Verification items for this drawing (mm, ordinates from the low corner). Coordinates: 2 decimals unless noted, no trailing zeros. Order: outer loops, then holes, each group sorted by start corner. A loop starts at its lowest first (then second) coordinate and runs counter-clockwise, first axis right, second up. Notation, with made-up numbers: M 35.25,30 L 91.25,30 A17 cw 91.25,62 Z; hole C -14,-40 d5. An arc over 180 degrees is marked long. Answer as a JSON object with one key per item and string values. Group by question number.
(1) Material ranges on line 1 (Z direction, x = 0.3, y = 78); line 2 (Z direction, x = 1.05, y = 45.5) (1 decimal); line 3 (Y direction, x = 1.3, z = 98), recorded low to high.
(2) Cross-section at D-D (y = 67.5). Enter the section's corners in (x, z).
(3) Cross-section at A-A (y = 122.5). Enter the section's corners in (x, z), plus the area to 3 significant figures.
(4) Cross-section at C-C (x = 0.6). Enter the section's corners in (y, z).
(5) Cross-section at B-B (z = 72.5). Enter the section's corners in (x, y).
(6) Gauge pin test, flat ends, axial feed: pin 1 Ø2 at (x, y) = (2.5, 65.5) entering from -Z; pin 2 Ø2 at (x, y) = (1, 64.5) entering from +Z; pin 3 Ø1 at (x, z) = (2, 47) entering from -Y. Record the tip position at first contact, or that the pin passes through.
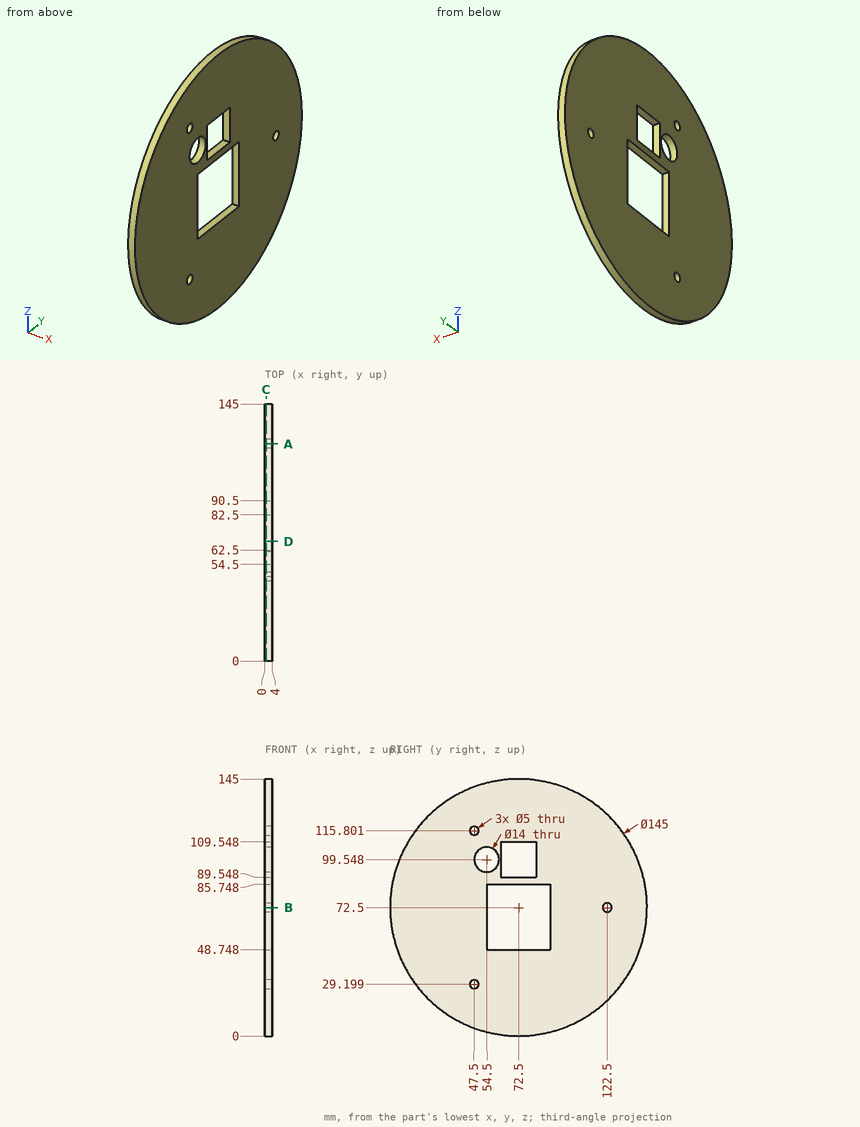
Taken from the geometry:
{
 "1": {"line 1": "z = 0.21 to 48.75, 85.75 to 89.55, 109.55 to 144.79", "line 2": "z = 5.2 to 27.7, 30.7 to 114.3, 117.3 to 139.8", "line 3": "y = 4.63 to 47.67, 61.33 to 62.5, 82.5 to 140.37"},
 "2": {"outline": "M 0,0.17 L 4,0.17 L 4,48.75 L 0,48.75 Z; M 0,85.75 L 4,85.75 L 4,89.55 L 0,89.55 Z; M 0,109.55 L 4,109.55 L 4,144.83 L 0,144.83 Z"},
 "3": {"outline": "M 0,20 L 4,20 L 4,70 L 0,70 Z; M 0,75 L 4,75 L 4,125 L 0,125 Z", "area": "400 mm²"},
 "4": {"outline": "C 72.5,72.5 d145; hole C 47.5,29.2 d5; hole C 47.5,115.8 d5; hole C 54.5,99.55 d14; hole M 54.5,48.75 L 90.5,48.75 L 90.5,85.75 L 54.5,85.75 Z; hole M 62.5,89.55 L 82.5,89.55 L 82.5,109.55 L 62.5,109.55 Z; hole C 122.5,72.5 d5"},
 "5": {"outline": "M 0,0 L 4,0 L 4,54.5 L 0,54.5 Z; M 0,90.5 L 4,90.5 L 4,120 L 0,120 Z; M 0,125 L 4,125 L 4,145 L 0,145 Z"},
 "6": {"pin 1": "stops at z = 0.25", "pin 2": "stops at z = 144.66", "pin 3": "stops at y = 4.45"}
}
